Work out the finished part from the listing and answer in its coordinate system (mm). A direction names the side the tool comes from. Round coordinates to 2 decimals unless told otherwise and drop trailing zeros. Loops run counter-clockwise (first coordinate to the right, second up) from the corner with the lowest first, then second, coordinate; pieces in that order, holes last. Notation, with made-up numbers: M -32,36 L -4,36 A9 cw -4,52 Z; hole C 58,84 d1. An arc over 180 degrees is marked long. One line per item, written item: value.
```python
from build123d import *

# Parameters (mm, degrees)
SKETCH2_R           = 4.25
BOSS_EXTRUDE1_DEPTH = 30
SKETCH3_R           = 11.25
SKETCH3_R_2         = 5.25
SKETCH3_R_3         = 4.25
CUT_EXTRUDE1_DEPTH  = 5
CUT_EXTRUDE2_START  = -5
SKETCH3_3_R         = 5.25
SKETCH3_3_R_2       = 4.25
CUT_EXTRUDE2_DEPTH  = 10.6
SKETCH4_R           = 2.4
CUT_EXTRUDE3_DEPTH  = 72.819217484


with BuildPart() as part:
    # Sketch2 → Boss-Extrude1 (new body)
    with BuildSketch(Plane(origin=(0, 0, 0), x_dir=(1, 0, 0), z_dir=(0, 1, 0))):
        with BuildLine():
            Line((0, 17), (0, -17))
            Line((0, -17), (5, -17))
            Line((5, -17), (5, -7))
            Line((5, -7), (44.04554885, -7))
            ThreePointArc((44.04554885, -7), (68, 0), (44.04554885, 7))
            Line((44.04554885, 7), (5, 7))
            Line((5, 7), (5, 17))
            Line((5, 17), (0, 17))
        make_face()
        with Locations(Location((55, 0, 0), (0, 0, 270))):
            Circle(SKETCH2_R, mode=Mode.SUBTRACT)
    extrude(amount=BOSS_EXTRUDE1_DEPTH)

    # Sketch3 → Cut-Extrude1 (cut)
    with BuildSketch(Plane.XZ):
        with Locations(Location((55, 0, 0), (0, 0, 270))):
            Circle(SKETCH3_R)
        with Locations((55, 0)):
            Circle(SKETCH3_R_2, mode=Mode.SUBTRACT)
        with Locations((55, 0)):
            Circle(SKETCH3_R_2)
        with Locations(Location((55, 0, 0), (0, 0, 270))):
            Circle(SKETCH3_R_3, mode=Mode.SUBTRACT)
    extrude(amount=-CUT_EXTRUDE1_DEPTH, mode=Mode.SUBTRACT)

    # Sketch3<3> → Cut-Extrude2 (cut)
    with BuildSketch(Plane.XZ.offset(CUT_EXTRUDE2_START)):
        with Locations(Location((55, 0, 0), (0, 0, 270))):
            Circle(SKETCH3_3_R)
        with Locations(Location((55, 0, 0), (0, 0, 270))):
            Circle(SKETCH3_3_R_2, mode=Mode.SUBTRACT)
    extrude(amount=-CUT_EXTRUDE2_DEPTH, mode=Mode.SUBTRACT)

    # Sketch4 → Cut-Extrude3 (cut, through all)
    with BuildSketch(Plane(origin=(5, 0, 0), x_dir=(0, 0, -1), z_dir=(1, 0, 0))):
        with Locations((12.17186788, 24.363439063)):
            Circle(SKETCH4_R)
        with Locations((12.17186788, 6.363439063)):
            Circle(SKETCH4_R)
        with Locations((-11.82813212, 6.363439063)):
            Circle(SKETCH4_R)
        with Locations((-11.82813212, 24.363439063)):
            Circle(SKETCH4_R)
    extrude(amount=-CUT_EXTRUDE3_DEPTH, mode=Mode.SUBTRACT)


solid = part.part
```
1) Find section C-C (z = 0). Give the vertices of the cut face in (x, y), then the cut area to 3 significant figures.
Check values:
outline: M 0,0 L 43.75,0 L 43.75,5 L 49.75,5 L 49.75,15.6 L 50.75,15.6 L 50.75,30 L 0,30 Z; M 59.25,15.6 L 60.25,15.6 L 60.25,5 L 66.25,5 L 66.25,0 L 68,0 L 68,30 L 59.25,30 Z
area: 1,690 mm2
2) Find section D-D (y = 14). Give the vertices of the cut face in (x, z).
Check values:
outline: M 0,-17 L 5,-17 L 5,-7 L 44.05,-7 A13 ccw long 44.05,7 L 5,7 L 5,17 L 0,17 Z; hole C 55,0 d10.5
3) The mould has two halves that part along Y. Classify faces 1 (the face through (34, 30, 0)), 2 (the face through (2.535, 4.234, -13.279)), 3 (the face through (50.85, 22.7, -0.92)): +Y half, -Y half, draft (parallel to the pull), parting line (faces both ways), or undercut.
Check values:
face 1: +Y half
face 2: undercut
face 3: draft
4) Find the intervals of material crossed by probe 1 along X at (y, z) = (26, 0); probe 2 along X at (y, z) = (2.85, 0); probe 3 along Y at (x, z) = (47, -5.5), in increasing order. Write a range as from..to.
Check values:
probe 1: 0..50.75, 59.25..68
probe 2: 0..43.75, 66.25..68
probe 3: 5..30
5) Find section B-B (y = 2.5). Give the vertices of the cut face in (x, z).
Check values:
outline: M 0,-17 L 5,-17 L 5,-7 L 44.05,-7 A13 ccw long 44.05,7 L 5,7 L 5,17 L 0,17 Z; hole C 55,0 d22.5
6) For faces 4 (the face through (5, 15, 12)), 5 (the face through (25, 15, -7)), 6 (the face through (51, 15.6, -2)), 7 (the face through (2.535, 26.743, 12.141)), determine the directions among +Z, -Z, +X, -X, +Y, -Y from which every point of the face is accessible in a straight line to the end or side of a thin tool.
Check values:
face 4: +Z, +Y, -Y
face 5: -Z, +Y, -Y
face 6: -Y
face 7: -X
7) Each of these flat-tipped pins is pushed along its axis until it touches: pin 1 (1 mm diameter, centred on y = 23, z = -7.5, fed in from +X); pin 2 (12 mm diameter, centred on x = 37.5, z = 0, fed in from -Y); pin 3 (15 mm diameter, centred on x = 25, y = 13.5, fed in from +Z); pin 4 (3 mm diameter, centred on y = 6.36, z = -12.17, fed in from +X). Where does it stop, or does it pass through?
Check values:
pin 1: x = 65.95
pin 2: y = 0
pin 3: z = 7
pin 4: x = 62.43
8) Find section A-A (x = 55). Give the vertices of the cut face in (y, z).
Check values:
outline: M 0,-13 L 30,-13 L 30,-4.25 L 15.6,-4.25 L 15.6,-5.25 L 5,-5.25 L 5,-11.25 L 0,-11.25 Z; M 0,11.25 L 5,11.25 L 5,5.25 L 15.6,5.25 L 15.6,4.25 L 30,4.25 L 30,13 L 0,13 Z
